Autodesk Inventor part; units mm, degrees
ref_plane "Work Plane1" through (7.366, 0, 0) normal (1, 0, 0) x (0, 1, 0)
ref_plane "XZ Plane" through (0, 0, 0) normal (0, 1, 0) x (-1, 0, 0)
ref_plane "XY Plane" through (0, 0, 0) normal (0, 0, 1) x (1, 0, 0)
sketch "Sketch1" plane through (0, 0, 0) normal (0, 0, 1) x (1, 0, 0)
  line L0 (0, 0) -> (13.716, 0)
  line L1 (13.716, 0) -> (13.716, 11.7856)
  line L2 (13.716, 11.7856) -> (0, 11.7856)
  line L3 (0, 11.7856) -> (0, 0)
  dimension "d0" = 13.716
  dimension "d1" = 11.7856
extrude "Extrusion1" add sketch "Sketch1" along normal blind 2.54
sketch "Sketch2" plane through (0, 0, 2.54) normal (0, 0, 1) x (1, 0, 0)
  line L0 (13.716, 0) -> (13.716, 11.7856)
  line L1 (13.716, 11.7856) -> (0, 11.7856)
  circle A0 centre (6.35, 5.8928) radius 3.4544
  dimension "d4" = 6.9088
  dimension "d5" = 7.366
  dimension "d6" = 11.7856
  dimension "d7" = 5.8928
extrude "Extrusion2" add sketch "Sketch2" along normal blind 8.001
thread "Thread1"
sketch "Sketch3" plane through (0, 0, 2.54) normal (0, 0, 1) x (1, 0, 0)
  circle A0 centre (6.35, 5.8928) radius 3.4544
  circle A1 centre (6.35, 5.8928) radius 4.826
  dimension "d12" = 9.652
extrude "Extrusion3" add sketch "Sketch3" along normal blind 0.381
chamfer "Chamfer1" distance 0.381 angle 45 1 edges at (2.8956, 5.8928, 10.541)
ref_plane "Work Plane1" through (7.366, 0, 0) normal (1, 0, 0) x (0, 1, 0)
sketch "Sketch4" plane through (7.366, 0, 0) normal (1, 0, 0) x (0, 1, 0)
  line L0 (11.7856, 0) -> (0, 0)
  line L1 (9.3472, 2.921) -> (2.4384, 2.921)
  line L2 (5.8928, 2.921) -> (5.8928, -2.4744)
  line L3 (9.3472, 2.921) -> (9.0932, 2.921)
  line L4 (9.0932, 2.921) -> (9.0932, 3.556)
  line L5 (9.0932, 3.556) -> (9.3472, 3.556)
  line L6 (9.3472, 3.556) -> (9.3472, 2.921)
  dimension "d19" = 0.254
  dimension "d20" = 0.635
revolve "Revolution1" cut sketch "Sketch4" angle 360 about axis through (7.366, 5.8928, 2.921) along (0, 0, -1)
sketch "Sketch5" plane through (6.35, 5.8928, 10.541) normal (0, 0, 1) x (1, 0, 0)
  circle A0 centre (0, 0) radius 4.826
  circle A1 centre (0, 0) radius 1.4986
  point P0 (-6.35, -5.8928)
  dimension "d22" = 2.9972
extrude "Extrusion4" cut sketch "Sketch5" against normal blind 1.016 contours A1
sketch "Sketch6" plane through (0, 0, 2.54) normal (0, 0, 1) x (1, 0, 0)
  line L0 (0, 0) -> (13.716, 0)
  line L1 (13.716, 11.7856) -> (0, 11.7856)
  line L2 (8.763, 0) -> (11.938, 0)
  line L3 (11.938, 0) -> (11.938, 1.143)
  line L4 (11.938, 1.143) -> (8.763, 1.143)
  line L5 (8.763, 1.143) -> (8.763, 0)
  line L6 (0.762, 0) -> (3.937, 0)
  line L7 (3.937, 0) -> (3.937, 1.143)
  line L8 (3.937, 1.143) -> (0.762, 1.143)
  line L9 (0.762, 1.143) -> (0.762, 0)
  line L10 (0.762, 11.7856) -> (3.937, 11.7856)
  line L11 (3.937, 11.7856) -> (3.937, 10.6426)
  line L12 (3.937, 10.6426) -> (0.762, 10.6426)
  line L13 (0.762, 10.6426) -> (0.762, 11.7856)
  line L14 (8.763, 11.7856) -> (11.938, 11.7856)
  line L15 (11.938, 11.7856) -> (11.938, 10.6426)
  line L16 (11.938, 10.6426) -> (8.763, 10.6426)
  line L17 (8.763, 10.6426) -> (8.763, 11.7856)
  circle A0 centre (6.35, 5.8928) radius 4.826
  arc A1 (6.8134, 3.2019) -> (3.704, 6.5668) centre (6.35, 5.8928) ccw
  circle A2 centre (6.35, 5.8928) radius 1.4859
  point P0 (11.938, 0.5715)
  point P1 (11.938, 11.2141)
  point P2 (0.762, 0.5715)
  point P3 (0.762, 11.2141)
  point P4 (2.3495, 10.6426)
  point P5 (10.3505, 10.6426)
  point P6 (2.3495, 1.143)
  point P7 (10.3505, 1.143)
  dimension "d25" = 3.175
  dimension "d26" = 3.175
  dimension "d27" = 3.175
  dimension "d28" = 3.175
  dimension "d29" = 13.716
  dimension "d30" = 11.176
  dimension "d32" = 1.143
  dimension "d33" = 1.143
  dimension "d34" = 4.826
  dimension "d35" = 0.762
extrude "Extrusion5" cut sketch "Sketch6" against normal blind 1.905 contours L9 L8 L7 L0 | L5 L4 L3 L0 | L15 L16 L17 L1 | L11 L12 L13 L1
sketch "Sketch7" plane through (0, 0, 0) normal (0, -1, 0) x (1, 0, 0)
  line L0 (3.937, 2.54) -> (3.937, 0.635)
  line L1 (3.937, 0.635) -> (0.762, 0.635)
  line L2 (0.762, 0.635) -> (0.762, 2.54)
  line L3 (0, 2.54) -> (0.762, 2.54)
  line L4 (0, 0) -> (0, 2.54)
  line L5 (0, 0) -> (13.716, 0)
  line L6 (11.938, 0.635) -> (8.763, 0.635)
  line L7 (8.763, 0.635) -> (8.763, 2.54)
  line L8 (3.937, 2.54) -> (8.763, 2.54)
  line L9 (11.6205, 0.635) -> (11.6205, 0)
  line L10 (8.763, 0.635) -> (11.938, 0.635)
  line L11 (9.0805, 0.635) -> (9.0805, 0)
  line L12 (13.716, 0) -> (0, 0)
  dimension "d38" = 3.175
  dimension "d39" = 2.54
  dimension "d40" = 0.3175
extrude "Extrusion6" cut sketch "Sketch7" against normal up to surface (1.143 mm away) contours L6 L9 L5 L11
sketch "Sketch8" plane through (0, 0, 0) normal (0, -1, 0) x (1, 0, 0)
  line L0 (3.937, 0.635) -> (0.762, 0.635)
  line L1 (0, 0) -> (9.0805, 0)
  line L2 (1.0795, 0.635) -> (3.6195, 0.635)
  line L3 (3.6195, 0.635) -> (3.6195, 0)
  line L4 (3.6195, 0) -> (1.0795, 0)
  line L5 (1.0795, 0) -> (1.0795, 0.635)
  dimension "d43" = 2.54
  dimension "d44" = 3.175
  dimension "d45" = 0.3175
extrude "Extrusion7" cut sketch "Sketch8" against normal up to surface (1.143 mm away)
sketch "Sketch9" plane through (0, 11.7856, 0) normal (0, 1, 0) x (1, 0, 0)
  line L0 (11.938, -0.635) -> (11.938, -2.54)
  line L1 (13.716, 0) -> (0, 0)
  line L2 (0.762, -0.635) -> (3.937, -0.635)
  line L3 (8.763, -2.54) -> (3.937, -2.54)
  line L4 (1.0795, -0.635) -> (3.6195, -0.635)
  line L5 (3.6195, -0.635) -> (3.6195, 0)
  line L6 (3.6195, 0) -> (1.0795, 0)
  line L7 (1.0795, 0) -> (1.0795, -0.635)
  line L8 (6.35, -2.54) -> (6.35, 1.5973)
  line L9 (11.6205, -0.635) -> (9.0805, -0.635)
  line L10 (9.0805, -0.635) -> (9.0805, 0)
  line L11 (9.0805, 0) -> (11.6205, 0)
  line L12 (11.6205, 0) -> (11.6205, -0.635)
  point P0 (12.7, 0)
  point P1 (11.938, -0.635)
  dimension "d48" = 2.54
  dimension "d49" = 3.175
  dimension "d50" = 0.3175
  dimension "d51" = 0.3175
extrude "Extrusion8" cut sketch "Sketch9" against normal up to surface (1.143 mm away)
equation "\"d7\" = 0.5 * d6"
equation "\"d40\" = -0.5 * d39 + 0.5 * d38"
equation "\"d45\" = -0.5 * d43 + 0.5 * d44"
equation "\"d50\" = -0.5 * d48 + 0.5 * d49"
properties part number "mtg flange"
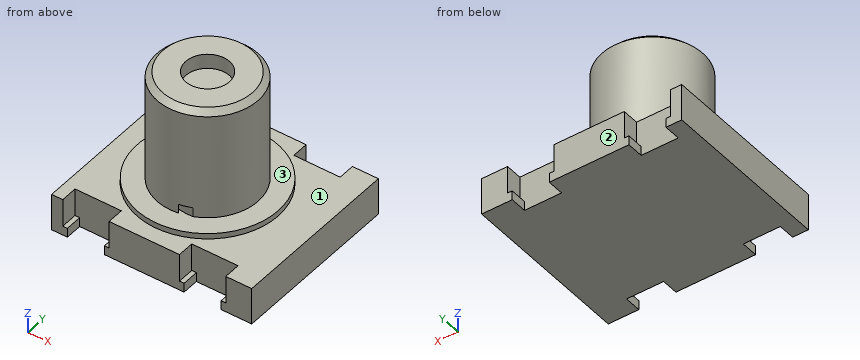
Design review of the part built by this model. Coordinates are the model's own, in mm. Face numbers are marked on the shaded views. A direction names the side the tool comes from. Coordinates: 2 decimals unless noted, no trailing zeros. Write each loop counter-clockwise with the first axis right and the second up, starting at its lowest first coordinate (ties: lowest second). Pieces come first, ordered by that corner, then holes.
1) Machinability: for the marked faces 1, 2 and 3, which of the approach directions +Z, -Z, +X, -X, +Y, -Y give a long, thin tool a straight path to every point of the face, cutting with its end or side? Answer none if there is none.
2) Insertion check: pin 1 (1.5 mm diameter, centred on y = 4, z = 4, fed in from -X); pin 2 (1.5 mm diameter, centred on y = 5.5, z = 4.5, fed in from -X); pin 3 (1.3 mm diameter, centred on y = 11.5, z = 2, fed in from -X); pin 4 (2 mm diameter, centred on y = 9, z = 8.5, fed in from +X). Each pin has a flat end and moves straight along its axis. Give the tip position at first contact, or say it passes through.
3) Add section A-A (x = 6.35). Write out the cut boundary in (y, z) (3 decimals), plus the area to 3 significant figures.
4) Add section B-B (z = 5.5). Write out the cut boundary in (x, y).
5) To check wall thickness, follow L1, parallel to Y at x = 6.35, z = 9.75; L2, parallel to Z at x = 0.5, y = 6.5; L3, parallel to Z at x = 9.75, y = 2.5. State the ranges of each line that lie inside material, in increasing order.
Check result:
1. face 1: +Z
1. face 2: +Z, -Z, +X, -X, +Y
1. face 3: none
2. pin 1: stops at x = 3.09
2. pin 2: stops at x = 2.9
2. pin 3: stops at x = 0
2. pin 4: stops at x = 9.09
3. outline: (0, 0) - (11.786, 0) - (11.786, 2.54) - (10.719, 2.54) - (10.719, 2.921) - (9.347, 2.921) - (9.347, 10.16) - (8.966, 10.541) - (7.391, 10.541) - (7.391, 9.525) - (4.394, 9.525) - (4.394, 10.541) - (2.819, 10.541) - (2.438, 10.16) - (2.438, 2.921) - (1.067, 2.921) - (1.067, 2.54) - (0, 2.54) - close; hole (2.591, 2.921) - (2.858, 2.921) - (2.858, 3.556) - (2.591, 3.556) - close; hole (8.928, 2.921) - (9.194, 2.921) - (9.194, 3.556) - (8.928, 3.556) - close
3. area: 82.7 mm2
4. outline: circle Ø6.91 at (6.35, 5.89)
5. L1: y = 2.44 to 4.39, 7.39 to 9.35
5. L2: z = 0 to 2.54
5. L3: z = 0 to 2.92
